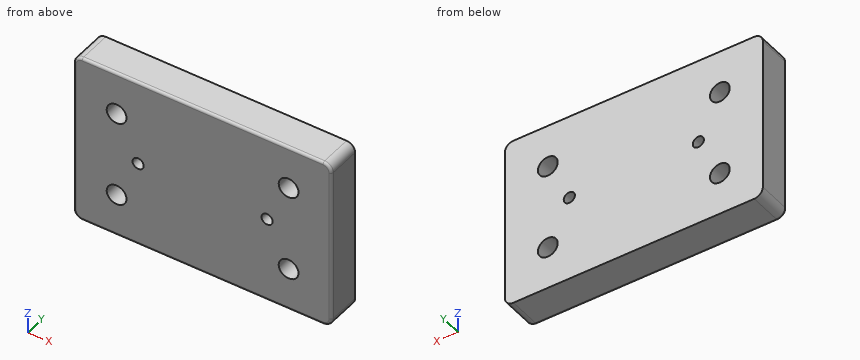
from build123d import *

# Parameters (mm, degrees)
SKETCH3_W           = 30
SKETCH3_H           = 20
SKETCH3_R           = 0.65
BOSS_EXTRUDE5_DEPTH = 4
CUT_EXTRUDE1_DEPTH  = 2
FILLET1_R           = 0.3
FILLET2_R           = 1
SKETCH10_R          = 1.15
SKETCH10_R_2        = 0.65
CUT_EXTRUDE3_DEPTH  = 10
FILLET3_R           = 1


with BuildPart() as part:
    # Sketch3 → Boss-Extrude5 (new body)
    with BuildSketch(Plane(origin=(0, 0, 0), x_dir=(1, 0, 0), z_dir=(0, 1, 0))):
        Rectangle(SKETCH3_W, SKETCH3_H)
        with Locations(Location((7.5, 0, 0), (0, 0, 270))):
            Circle(SKETCH3_R, mode=Mode.SUBTRACT)
        with Locations(Location((-7.5, 0, 0), (0, 0, 90))):
            Circle(SKETCH3_R, mode=Mode.SUBTRACT)
    extrude(amount=BOSS_EXTRUDE5_DEPTH)

    # Sketch6 → Cut-Extrude1 (cut)
    with BuildSketch(Plane(origin=(0, 4, 0), x_dir=(1, 0, 0), z_dir=(0, 1, 0))):
        with BuildLine():
            Line((-8.85, 5), (-10, 5))
            Line((-10, 5), (-10, 3.85))
            ThreePointArc((-10, 3.85), (-9.186827202, 4.186827202), (-8.85, 5))
        make_face()
        with BuildLine():
            Line((-10, 3.85), (-10, 5))
            Line((-10, 5), (-8.85, 5))
            ThreePointArc((-8.85, 5), (-10.813172798, 5.813172798), (-10, 3.85))
        make_face()
        with BuildLine():
            ThreePointArc((11.15, 5), (10, 6.15), (8.85, 5))
            Line((8.85, 5), (10, 5))
            Line((10, 5), (10, 3.85))
            ThreePointArc((10, 3.85), (10.813172798, 4.186827202), (11.15, 5))
        make_face()
        with BuildLine():
            Line((10, 5), (8.85, 5))
            ThreePointArc((8.85, 5), (9.186827202, 4.186827202), (10, 3.85))
            Line((10, 3.85), (10, 5))
        make_face()
        with BuildLine():
            ThreePointArc((10, -3.85), (9.186827202, -4.186827202), (8.85, -5))
            Line((8.85, -5), (10, -5))
            Line((10, -5), (10, -3.85))
        make_face()
        with BuildLine():
            Line((10, -5), (8.85, -5))
            ThreePointArc((8.85, -5), (10, -6.15), (11.15, -5))
            ThreePointArc((11.15, -5), (10.813172798, -4.186827202), (10, -3.85))
            Line((10, -3.85), (10, -5))
        make_face()
        with BuildLine():
            ThreePointArc((-8.85, -5), (-9.186827202, -4.186827202), (-10, -3.85))
            Line((-10, -3.85), (-10, -5))
            Line((-10, -5), (-8.85, -5))
        make_face()
        with BuildLine():
            Line((-10, -5), (-10, -3.85))
            ThreePointArc((-10, -3.85), (-10.813172798, -5.813172798), (-8.85, -5))
            Line((-8.85, -5), (-10, -5))
        make_face()
    extrude(amount=-CUT_EXTRUDE1_DEPTH, mode=Mode.SUBTRACT)

    # Fillet1
    fillet1_edges = [part.edges().sort_by_distance(p)[0] for p in [
        (0, 0, 10),
        (-15, 0, 0),
        (0, 0, -10),
        (15, 0, 0),
    ]]
    fillet(fillet1_edges, radius=FILLET1_R)

    # Fillet2
    # the kernel refuses this fillet: 1 mm, written as the material it takes off along each edge
    with BuildSketch(Plane(origin=(14, 0, 9), x_dir=(1, 0, 0), z_dir=(0, 0, -1))) as fillet2_piece_1:
        with BuildLine():
            CenterArc((0.7, -0.3), 0.3, 0, 90)
            Line((1, -0.3), (1, 0))
            Line((1, 0), (0.7, 0))
        make_face()
    revolve(axis=Axis((14, 0, 9), (0, -1, 0)), revolution_arc=90, mode=Mode.SUBTRACT)
    with BuildSketch(Plane(origin=(14, 0, -9), x_dir=(0, 0, -1), z_dir=(-1, 0, 0))) as fillet2_piece_2:
        with BuildLine():
            CenterArc((0.7, -0.3), 0.3, 0, 90)
            Line((1, -0.3), (1, 0))
            Line((1, 0), (0.7, 0))
        make_face()
    revolve(axis=Axis((14, 0, -9), (0, -1, 0)), revolution_arc=90, mode=Mode.SUBTRACT)
    with BuildSketch(Plane(origin=(15, 0, 10), x_dir=(-1, 0, 0), z_dir=(0, 1, 0)), Plane(origin=(15, 0, -10), x_dir=(0, 0, 1), z_dir=(0, 1, 0))) as fillet2_piece_3:
        with BuildLine():
            CenterArc((FILLET2_R, -FILLET2_R), FILLET2_R, 90, 90)
            Line((0, -FILLET2_R), (0, 0))
            Line((0, 0), (FILLET2_R, 0))
        make_face()
    extrude(amount=6.5, mode=Mode.SUBTRACT)

    # Sketch10 → Cut-Extrude3 (cut)
    with BuildSketch(Plane(origin=(0, 2, 0), x_dir=(1, 0, 0), z_dir=(0, 1, 0))):
        with Locations(Location((10, -5, 0), (0, 0, 270))):
            Circle(SKETCH10_R)
        with Locations(Location((-7.5, 0, 0), (0, 0, 90))):
            Circle(SKETCH10_R_2)
        with Locations(Location((-10, 5, 0), (0, 0, 270))):
            Circle(SKETCH10_R)
        with Locations(Location((7.5, 0, 0), (0, 0, 270))):
            Circle(SKETCH10_R_2)
        with Locations(Location((10, 5, 0), (0, 0, 270))):
            Circle(SKETCH10_R)
        with Locations(Location((-10, -5, 0), (0, 0, 270))):
            Circle(SKETCH10_R)
    extrude(amount=-CUT_EXTRUDE3_DEPTH, mode=Mode.SUBTRACT)

    # Fillet3
    # the kernel refuses this fillet: 1 mm, written as the material it takes off along each edge
    with BuildSketch(Plane(origin=(-14, 0, 9), x_dir=(0, 0, 1), z_dir=(1, 0, 0))) as fillet3_piece_1:
        with BuildLine():
            CenterArc((0.7, -0.3), 0.3, 0, 90)
            Line((1, -0.3), (1, 0))
            Line((1, 0), (0.7, 0))
        make_face()
    revolve(axis=Axis((-14, 0, 9), (0, -1, 0)), revolution_arc=90, mode=Mode.SUBTRACT)
    with BuildSketch(Plane(origin=(-14, 0, -9), x_dir=(-1, 0, 0), z_dir=(0, 0, 1))) as fillet3_piece_2:
        with BuildLine():
            CenterArc((0.7, -0.3), 0.3, 0, 90)
            Line((1, -0.3), (1, 0))
            Line((1, 0), (0.7, 0))
        make_face()
    revolve(axis=Axis((-14, 0, -9), (0, -1, 0)), revolution_arc=90, mode=Mode.SUBTRACT)
    with BuildSketch(Plane(origin=(-15, 0, 10), x_dir=(1, 0, 0), z_dir=(0, 1, 0)), Plane(origin=(-15, 0, -10), x_dir=(0, 0, 1), z_dir=(0, 1, 0))) as fillet3_piece_3:
        with BuildLine():
            CenterArc((FILLET3_R, FILLET3_R), FILLET3_R, 180, 90)
            Line((0, FILLET3_R), (0, 0))
            Line((0, 0), (FILLET3_R, 0))
        make_face()
    extrude(amount=6.5, mode=Mode.SUBTRACT)


solid = part.part
Geometry: final body of the model. Coordinates: model frame, mm. Give positions to 0.01 mm unless a question says otherwise; leave off trailing zeros. Write each loop counter-clockwise with the first axis right and the second up, starting at its lowest first coordinate (ties: lowest second). Pieces come first, ordered by that corner, then holes. Notation, with made-up numbers: M -4.75,82.5 L 27.25,82.5 A23 cw 27.25,114.5 Z; hole C 67,5 d11. An arc over 180 degrees is marked long. Answer in a Markdown table with one row per item. Add a question column.
(1) First-contact query: pin 1 (1.8 mm diameter, centred on x = 10, z = -5, fed in from +Y); pin 2 (3.5 mm diameter, centred on x = -10, z = 5, fed in from +Y). Flat tips, straight axial feed; report the tip coordinate or a pass-through.
(2) Section B-B on y = 2.95. Return loops of the section in (x, z).
(3) Ray query, line 1 (Z direction, x = -10, y = 2.6); line 2 (X direction, y = 2.1, z = -5); line 3 (X direction, y = 1.6, z = 0). Return the intervals inside material, ascending.
Result set:
| question | item | result |
|---|---|---|
| 1 | pin 1 | passes through |
| 1 | pin 2 | stops at y = 4 |
| 2 | outline | M -15,-9 A1 ccw -14,-10 L 14,-10 A1 ccw 15,-9 L 15,9 A1 ccw 14,10 L -14,10 A1 ccw -15,9 Z; hole C -10,-5 d2.3; hole C -10,5 d2.3; hole C -7.5,0 d1.3; hole C 7.5,0 d1.3; hole C 10,-5 d2.3; hole C 10,5 d2.3 |
| 3 | line 1 | z = -10 to -6.15, -3.85 to 3.85, 6.15 to 10 |
| 3 | line 2 | x = -15 to -11.15, -8.85 to 8.85, 11.15 to 15 |
| 3 | line 3 | x = -15 to -8.15, -6.85 to 6.85, 8.15 to 15 |
